Geometry: final body of the model. Coordinates: model frame, mm. Give positions to 0.01 mm unless a question says otherwise; leave off trailing zeros. Write each loop counter-clockwise with the first axis right and the second up, starting at its lowest first coordinate (ties: lowest second). Pieces come first, ordered by that corner, then holes. Notation, with made-up numbers: M 46,63 L 81,63 A19 ccw 81,96 Z; hole C 3.25,70.5 d1. An arc over 180 degrees is marked long. Use a Markdown table: item, result. Add a question column.
(1) Cut plane B-B (x = 143). Output: boundary loops of the cut face in (y, z) (3 decimals), plus the area to 4 significant figures.
(2) Cut plane C-C (z = 1.1). State how many separate pieces and enclosed holes the cut face has, plus the area to 3 significant figures.
(3) Material intervals for L1, parallel to X at y = -13, z = 1.05 (3 decimals); L2, parallel to Y at x = 128, z = 0.9 (3 decimals); L3, parallel to Y at x = 139.5, z = 1.2 (3 decimals), sorted ascending.
(4) Cut plane A-A (y = -14). Output: boundary loops of the cut face in (x, z) (3 decimals).
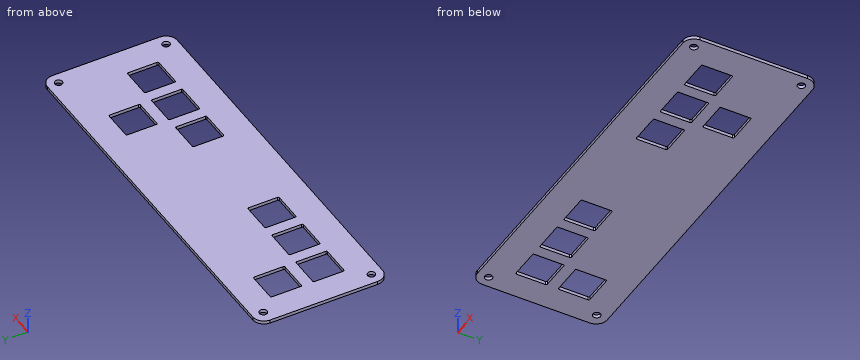
Autodesk Fusion 360 part; units mm, degrees
sketch "plate" plane through (0, 0, 0) normal (0, 0, 1) x (1, 0, 0)
  line L0 (3.025, -2.525) -> (16.025, -2.525)
  line L1 (3.025, -16.525) -> (16.025, -16.525)
  line L2 (2.525, -3.025) -> (2.525, -16.025)
  line L3 (16.525, -3.025) -> (16.525, -16.025)
  arc A0 (3.025, -2.525) -> (2.525, -3.025) centre (3.025, -3.025) ccw
  arc A1 (16.525, -3.025) -> (16.025, -2.525) centre (16.025, -3.025) ccw
  arc A2 (2.525, -16.025) -> (3.025, -16.525) centre (3.025, -16.025) ccw
  arc A3 (16.025, -16.525) -> (16.525, -16.025) centre (16.025, -16.025) ccw
  line L4 (117.325, -2.525) -> (130.325, -2.525)
  line L5 (117.325, -16.525) -> (130.325, -16.525)
  line L6 (116.825, -3.025) -> (116.825, -16.025)
  line L7 (130.825, -3.025) -> (130.825, -16.025)
  arc A4 (117.325, -2.525) -> (116.825, -3.025) centre (117.325, -3.025) ccw
  arc A5 (130.825, -3.025) -> (130.325, -2.525) centre (130.325, -3.025) ccw
  arc A6 (116.825, -16.025) -> (117.325, -16.525) centre (117.325, -16.025) ccw
  arc A7 (130.325, -16.525) -> (130.825, -16.025) centre (130.325, -16.025) ccw
  line L8 (3.025, -21.575) -> (16.025, -21.575)
  line L9 (3.025, -35.575) -> (16.025, -35.575)
  line L10 (2.525, -22.075) -> (2.525, -35.075)
  line L11 (16.525, -22.075) -> (16.525, -35.075)
  arc A8 (3.025, -21.575) -> (2.525, -22.075) centre (3.025, -22.075) ccw
  arc A9 (16.525, -22.075) -> (16.025, -21.575) centre (16.025, -22.075) ccw
  arc A10 (2.525, -35.075) -> (3.025, -35.575) centre (3.025, -35.075) ccw
  arc A11 (16.025, -35.575) -> (16.525, -35.075) centre (16.025, -35.075) ccw
  line L12 (22.075, -21.575) -> (35.075, -21.575)
  line L13 (22.075, -35.575) -> (35.075, -35.575)
  line L14 (21.575, -22.075) -> (21.575, -35.075)
  line L15 (35.575, -22.075) -> (35.575, -35.075)
  arc A12 (22.075, -21.575) -> (21.575, -22.075) centre (22.075, -22.075) ccw
  arc A13 (35.575, -22.075) -> (35.075, -21.575) centre (35.075, -22.075) ccw
  arc A14 (21.575, -35.075) -> (22.075, -35.575) centre (22.075, -35.075) ccw
  arc A15 (35.075, -35.575) -> (35.575, -35.075) centre (35.075, -35.075) ccw
  line L16 (41.125, -21.575) -> (54.125, -21.575)
  line L17 (41.125, -35.575) -> (54.125, -35.575)
  line L18 (40.625, -22.075) -> (40.625, -35.075)
  line L19 (54.625, -22.075) -> (54.625, -35.075)
  arc A16 (41.125, -21.575) -> (40.625, -22.075) centre (41.125, -22.075) ccw
  arc A17 (54.625, -22.075) -> (54.125, -21.575) centre (54.125, -22.075) ccw
  arc A18 (40.625, -35.075) -> (41.125, -35.575) centre (41.125, -35.075) ccw
  arc A19 (54.125, -35.575) -> (54.625, -35.075) centre (54.125, -35.075) ccw
  line L20 (98.275, -21.575) -> (111.275, -21.575)
  line L21 (98.275, -35.575) -> (111.275, -35.575)
  line L22 (97.775, -22.075) -> (97.775, -35.075)
  line L23 (111.775, -22.075) -> (111.775, -35.075)
  arc A20 (98.275, -21.575) -> (97.775, -22.075) centre (98.275, -22.075) ccw
  arc A21 (111.775, -22.075) -> (111.275, -21.575) centre (111.275, -22.075) ccw
  arc A22 (97.775, -35.075) -> (98.275, -35.575) centre (98.275, -35.075) ccw
  arc A23 (111.275, -35.575) -> (111.775, -35.075) centre (111.275, -35.075) ccw
  line L24 (117.325, -21.575) -> (130.325, -21.575)
  line L25 (117.325, -35.575) -> (130.325, -35.575)
  line L26 (116.825, -22.075) -> (116.825, -35.075)
  line L27 (130.825, -22.075) -> (130.825, -35.075)
  arc A24 (117.325, -21.575) -> (116.825, -22.075) centre (117.325, -22.075) ccw
  arc A25 (130.825, -22.075) -> (130.325, -21.575) centre (130.325, -22.075) ccw
  arc A26 (116.825, -35.075) -> (117.325, -35.575) centre (117.325, -35.075) ccw
  arc A27 (130.325, -35.575) -> (130.825, -35.075) centre (130.325, -35.075) ccw
  line L28 (136.375, -21.575) -> (149.375, -21.575)
  line L29 (136.375, -35.575) -> (149.375, -35.575)
  line L30 (135.875, -22.075) -> (135.875, -35.075)
  line L31 (149.875, -22.075) -> (149.875, -35.075)
  arc A28 (136.375, -21.575) -> (135.875, -22.075) centre (136.375, -22.075) ccw
  arc A29 (149.875, -22.075) -> (149.375, -21.575) centre (149.375, -22.075) ccw
  arc A30 (135.875, -35.075) -> (136.375, -35.575) centre (136.375, -35.075) ccw
  arc A31 (149.375, -35.575) -> (149.875, -35.075) centre (149.375, -35.075) ccw
  line L32 (-9.515, 9.515) -> (162.885, 9.515)
  line L33 (162.885, 9.515) -> (162.885, -48.585)
  line L34 (162.885, -48.585) -> (-9.515, -48.585)
  line L35 (-9.515, -48.585) -> (-9.515, 9.515)
  circle A32 centre (-4, 4.515) radius 1.7
  circle A33 centre (157.885, 4.515) radius 1.7
  circle A34 centre (157.885, -43.585) radius 1.7
  circle A35 centre (-4.515, -43.585) radius 1.7
  dimension "d1" = 172.4
  dimension "d2" = 58.1
  dimension "d3" = 12.04
  dimension "d4" = 12.04
  dimension "d5" = 3.4
  dimension "d6" = 5
  dimension "d7" = 5.515
  dimension "d8" = 3.4
  dimension "d9" = 5
  dimension "d10" = 5
  dimension "d11" = 3.4
  dimension "d12" = 5
  dimension "d13" = 5
  dimension "d14" = 3.4
  dimension "d15" = 5
  dimension "d16" = 5
extrude "Extrude1" add sketch "plate" along normal blind 1.5
fillet "Fillet1" radius 5 4 edges at (162.885, -48.585, 0.75) (162.885, 9.515, 0.75) (-9.515, 9.515, 0.75) (-9.515, -48.585, 0.75)
Answer list:
| question | item | result |
|---|---|---|
| 1 | outline | M -48.585,0 L -35.575,0 L -35.575,1.5 L -48.585,1.5 Z; M -21.575,0 L 9.515,0 L 9.515,1.5 L -21.575,1.5 Z |
| 1 | area | 66.15 mm² |
| 2 | separate pieces | 1 |
| 2 | enclosed holes | 12 |
| 2 | area | 8,390 mm² |
| 3 | L1 | -9.515 to 2.525, 16.525 to 116.825, 130.825 to 162.885 |
| 3 | L2 | -48.585 to -35.575, -21.575 to -16.525, -2.525 to 9.515 |
| 3 | L3 | -48.585 to -35.575, -21.575 to 9.515 |
| 4 | outline | M -9.515,0 L 2.525,0 L 2.525,1.5 L -9.515,1.5 Z; M 16.525,0 L 116.825,0 L 116.825,1.5 L 16.525,1.5 Z; M 130.825,0 L 162.885,0 L 162.885,1.5 L 130.825,1.5 Z |
